from build123d import *

# Parameters (mm, degrees)
RESSALTO_EXTRUS_O1_DEPTH = 2
FILETE1_R                = 2


with BuildPart() as part:
    # Esboço1 → Ressalto-extrusão1 (new body)
    with BuildSketch(Plane.XY):
        Polygon((-7.5, 12.5), (-14.5, 12.5), (-14.5, 7.5), (-19, 7.5), (-22.5, -12.5), (22.5, -12.5), (19, 7.5), (14.5, 7.5), (14.5, 12.5), (7.5, 12.5), (7.5, 7.5), (3, 7.5), (0, -7.5), (-3, 7.5), (-7.5, 7.5), align=None)
        with BuildLine():
            ThreePointArc((-12, 0.5), (-11, 1.5), (-10, 0.5))
            Line((-10, 0.5), (-10, -9.5))
            ThreePointArc((-10, -9.5), (-11, -10.5), (-12, -9.5))
            Line((-12, -9.5), (-12, 0.5))
        make_face(mode=Mode.SUBTRACT)
        with BuildLine():
            Line((10, -9.5), (10, 0.5))
            ThreePointArc((10, 0.5), (11, 1.5), (12, 0.5))
            Line((12, 0.5), (12, -9.5))
            ThreePointArc((12, -9.5), (11, -10.5), (10, -9.5))
        make_face(mode=Mode.SUBTRACT)
    extrude(amount=RESSALTO_EXTRUS_O1_DEPTH)

    # Filete1
    filete1_edges = [part.edges().sort_by_distance(p)[0] for p in [
        (-22.5, -12.5, 1),
        (-19, 7.5, 1),
        (-14.5, 12.5, 1),
        (-7.5, 12.5, 1),
        (-3, 7.5, 1),
        (0, -7.5, 1),
        (7.5, 12.5, 1),
        (14.5, 12.5, 1),
        (19, 7.5, 1),
        (22.5, -12.5, 1),
    ]]
    fillet(filete1_edges, radius=FILETE1_R)


solid = part.part
Check sheet for the modelled part. Datum: model origin and axes. Units: mm. A direction names the side the tool comes from. Give positions to 0.01 mm unless a question says otherwise; leave off trailing zeros. Write each loop counter-clockwise with the first axis right and the second up, starting at its lowest first coordinate (ties: lowest second). Pieces come first, ordered by that corner, then holes. Notation, with made-up numbers: (-1, 72) -> (9, 72) arc R12 cw to (9, 85) -> close; hole circle Ø7 at (45.5, 79.5). An arc over 180 degrees is marked (long way). Use one line per item in the form item = value. Start each with the question number.
1. Go/stop test with flat-tipped pins: P1, Ø1, axis at x = 15, y = -7.5, coming from the -Z side; P2, Ø3, axis at x = 2.5, y = 10, coming from the -Z side; P3, Ø0.6, axis at y = -4, z = 0.5, coming from the +X side (3 decimals); P4, Ø0.6, axis at x = -6.5, z = 1.5, coming from the +Y side. Record where each tip stops, or that it passes through.
2. Section check A-A (x = 11). Record the cut outline in (y, z).
3. Thickness scan on line 1 along Y through (x, z) = (11, 0.75); line 2 along X through (y, z) = (9.75, 1.5); line 3 along X through (y, z) = (-3.5, 1.8) (3 decimals). Record the ranges inside material, lowest first. Write a range as from..to.
4. Access from +Z, -Z, +X, -X, +Y, -Y to the whole of each face (thin tool, end or side, straight path). Record for faces 1 (the flat face through (14.5, 9, 1)), 2 (the flat face through (11, 12.5, 1)), 3 (the flat face through (0, -3, 0)), 4 (the flat face through (7.5, 9, 1)), 5 (the flat face through (-14.5, 9, 1)).
5. Mould release check, pull along Y, two halves, no side actions. Record for faces 6 (the flat face through (-12, -5, 1)), 7 (the flat face through (-11, 12.5, 1)), 8 (the flat face through (0, -12.5, 1)), 9 (the cylindrical face through (11, 1.5, 1)): pulls with the +Y half, pulls with the -Y half, needs draft (parallel to the pull), parting line crosses it, or undercut.
6. Section check B-B (y = -7.5). Record the cut outline in (x, z) (3 decimals), and give its area (3 significant figures).
7. Section check D-D (y = 4.25). Record the cut outline in (x, z).
8. Section check C-C (z = 0.4). Count the separate pieces of the cut face and the enclosed holes in it, and give its area (3 significant figures).
Conclusion:
q1.P1 = 0
q1.P2 = through
q1.P3 = 21.065
q1.P4 = 7.5
q2.outline = (-12.5, 0) -> (-10.5, 0) -> (-10.5, 2) -> (-12.5, 2) -> close; (1.5, 0) -> (12.5, 0) -> (12.5, 2) -> (1.5, 2) -> close
q3.line_1 = -12.5..-10.5, 1.5..12.5
q3.line_2 = -14.5..-7.5, 7.5..14.5
q3.line_3 = -20.925..-12, -10..10, 12..20.925
q4.face_1 = +Z, -Z, +X, +Y
q4.face_2 = +Z, -Z, +X, -X, +Y
q4.face_3 = -Z, +X, -X, +Y, -Y
q4.face_4 = +Z, -Z, +Y
q4.face_5 = +Z, -Z, -X, +Y
q5.face_6 = undercut
q5.face_7 = pulls with the +Y half
q5.face_8 = pulls with the -Y half
q5.face_9 = undercut
q6.outline = (-21.625, 0) -> (-12, 0) -> (-12, 2) -> (-21.625, 2) -> close; (-10, 0) -> (10, 0) -> (10, 2) -> (-10, 2) -> close; (12, 0) -> (21.625, 0) -> (21.625, 2) -> (12, 2) -> close
q6.area = 78.5 mm²
q7.outline = (-19.57, 0) -> (-2.35, 0) -> (-2.35, 2) -> (-19.57, 2) -> close; (2.35, 0) -> (19.57, 0) -> (19.57, 2) -> (2.35, 2) -> close
q8.separate_pieces = 1
q8.enclosed_holes = 2
q8.area = 816 mm²
